Check sheet for the modelled part. Datum: model origin and axes. Units: mm. A direction names the side the tool comes from. Round coordinates to 2 decimals unless told otherwise and drop trailing zeros. Write each loop counter-clockwise with the first axis right and the second up, starting at its lowest first coordinate (ties: lowest second). Pieces come first, ordered by that corner, then holes. Notation, with made-up numbers: (50.5, 64.5) -> (71.5, 64.5) arc R9 ccw to (71.5, 78.5) -> close; hole circle Ø3 at (-25.75, -31.5). An arc over 180 degrees is marked (long way). Answer as a JSON object with one key per item and string values. Group by question number.
```python
from build123d import *

# Parameters (mm, degrees)
SKETCH1_W                                       = 75
SKETCH1_H                                       = 24
BOSS_EXTRUDE1_DEPTH                             = 24
SKETCH2_W                                       = 20
SKETCH2_H                                       = 12
CUT_EXTRUDE1_DEPTH                              = 24
FILLET1_START                                   = -1
FILLET1_DEPTH                                   = 26
FILLET1_2_DEPTH                                 = 24
CSK_FOR_M4_FLAT_HEAD_MACHINE_SCREW1_D           = 4.5
CSK_FOR_M4_FLAT_HEAD_MACHINE_SCREW1_CSINK_D     = 9.4
CSK_FOR_M4_FLAT_HEAD_MACHINE_SCREW1_CSINK_ANGLE = 90


with BuildPart() as part:
    # Sketch1 → Boss-Extrude1 (new body)
    with BuildSketch(Plane(origin=(0, 0, 0), x_dir=(0, 0, -1), z_dir=(1, 0, 0))):
        Rectangle(SKETCH1_W, SKETCH1_H)
    extrude(amount=BOSS_EXTRUDE1_DEPTH)

    # Sketch2 → Cut-Extrude1 (cut)
    with BuildSketch(Plane(origin=(24, 0, 0), x_dir=(0, 0, -1), z_dir=(1, 0, 0))):
        with Locations((-27.5, 6)):
            Rectangle(SKETCH2_W, SKETCH2_H)
    cut_extrude1 = extrude(amount=-CUT_EXTRUDE1_DEPTH, mode=Mode.SUBTRACT)

    # Fillet1: read off the stored shape, not the designer's step
    # Fillet1 outline → Fillet1 (cut)
    with BuildSketch(Plane.YZ.offset(FILLET1_START)):
        with BuildLine():
            Line((12, 17.5), (6, 17.5))
            ThreePointArc((6, 17.5), (10.242640687, 15.742640687), (12, 11.5))
            Line((12, 11.5), (12, 17.5))
        make_face()
    fillet1 = extrude(amount=FILLET1_DEPTH, mode=Mode.SUBTRACT)

    # Fillet1 2 outline → Fillet1 2 (add)
    with BuildSketch(Plane.YZ):
        with BuildLine():
            Line((0, 17.5), (6, 17.5))
            ThreePointArc((6, 17.5), (1.757359313, 19.257359313), (0, 23.5))
            Line((0, 23.5), (0, 17.5))
        make_face()
    fillet1_2 = extrude(amount=FILLET1_2_DEPTH)

    # CSK for M4 Flat Head Machine Screw1 (through all)
    with Locations(Plane(origin=(0, 0, 0), x_dir=(1, 0, 0), z_dir=(0, 1, 0))):
        with Locations((6, -28.5), (18, -28.702489343)):
            csk_for_m4_flat_head_machine_screw1 = CounterSinkHole(CSK_FOR_M4_FLAT_HEAD_MACHINE_SCREW1_D / 2, CSK_FOR_M4_FLAT_HEAD_MACHINE_SCREW1_CSINK_D / 2, counter_sink_angle=CSK_FOR_M4_FLAT_HEAD_MACHINE_SCREW1_CSINK_ANGLE)

    # Mirror1: Cut-Extrude1, Fillet1, Fillet1 2, CSK for M4 Flat Head Machine Screw1 across plane
    add(cut_extrude1.mirror(Plane.XY), mode=Mode.SUBTRACT)
    add(fillet1.mirror(Plane.XY), mode=Mode.SUBTRACT)
    add(fillet1_2.mirror(Plane.XY))
    add(csk_for_m4_flat_head_machine_screw1.mirror(Plane.XY), mode=Mode.SUBTRACT)


solid = part.part
```
(1) Scan lines: line 1 along Z through (x, y) = (6, -9); line 2 along Z through (x, y) = (18, -8); line 3 along Z through (x, y) = (22.75, 7). Record each from-to range of solid material in increasing order.
(2) Section check C-C on z = 16.5. Record the cut outline in (x, y), then the cut area to 3 significant figures.
(3) Section check B-B on y = -7.75. Record the cut outline in (x, z), then the cut area to 3 significant figures.
(4) Access from +Z, -Z, +X, -X, +Y, -Y to the whole of each face (thin tool, end or side, straight path). Record for faces 1 (the flat face through (12, -6, -37.5)), 2 (the flat face through (12, 0, -32)).
(5) Go/stop test with flat-tipped pins: pin 1 Ø2.5 at (x, z) = (18, -28.7) entering from +Y; pin 2 Ø11 at (x, z) = (15, 29.5) entering from +Y; pin 3 Ø1.5 at (x, y) = (19.5, 9.5) entering from -Z. Record where each tip stops, or that it passes through.
(6) Section check D-D on y = -1.5. Record the cut outline in (x, z), then the cut area to 3 significant figures.
(7) Release check for a two-part mould opening along X. For faces 3 (the flat face through (12, 0, 32)), 4 (the conical face through (15.81, -2.33, 29.61)), 5 (the flat face through (24, -3, -1)) record: pulls with the +X half, pulls with the -X half, needs draft (parallel to the pull), parting line crosses it, or undercut.
(8) Section check A-A on x = 18. Record the cut outline in (y, z).
Data:
{
 "1": {"line 1": "z = -37.5 to -30.75, -26.25 to 26.25, 30.75 to 37.5", "line 2": "z = -37.5 to -30.95, -26.45 to 26.45, 30.95 to 37.5", "line 3": "z = -17.42 to 17.42"},
 "2": {"outline": "(0, -12) -> (24, -12) -> (24, 9.32) -> (0, 9.32) -> close", "area": "512 mm²"},
 "3": {"outline": "(0, -37.5) -> (24, -37.5) -> (24, 37.5) -> (0, 37.5) -> close; hole circle Ø4.5 at (6, -28.5); hole circle Ø4.5 at (6, 28.5); hole circle Ø4.5 at (18, -28.7); hole circle Ø4.5 at (18, 28.7)", "area": "1,740 mm²"},
 "4": {"face 1": "-Z, +X, -X, +Y, -Y", "face 2": "-Z, +X, -X, +Y"},
 "5": {"pin 1": "passes through", "pin 2": "stops at y = 0", "pin 3": "stops at z = -16.83"},
 "6": {"outline": "(0, -37.5) -> (24, -37.5) -> (24, 37.5) -> (0, 37.5) -> close; hole circle Ø6.4 at (6, -28.5); hole circle Ø6.4 at (6, 28.5); hole circle Ø6.4 at (18, -28.7); hole circle Ø6.4 at (18, 28.7)", "area": "1,670 mm²"},
 "7": {"face 3": "needs draft", "face 4": "undercut", "face 5": "pulls with the +X half"},
 "8": {"outline": "(-12, -37.5) -> (0, -37.5) -> (0, -33.4) -> (-2.45, -30.95) -> (-12, -30.95) -> close; (-12, -26.45) -> (-2.45, -26.45) -> (0, -24) -> (0, -23.5) arc R6 cw to (6, -17.5) arc R6 ccw to (12, -11.5) -> (12, 11.5) arc R6 ccw to (6, 17.5) arc R6 cw to (0, 23.5) -> (0, 24) -> (-2.45, 26.45) -> (-12, 26.45) -> close; (-12, 30.95) -> (-2.45, 30.95) -> (0, 33.4) -> (0, 37.5) -> (-12, 37.5) -> close"}
}
